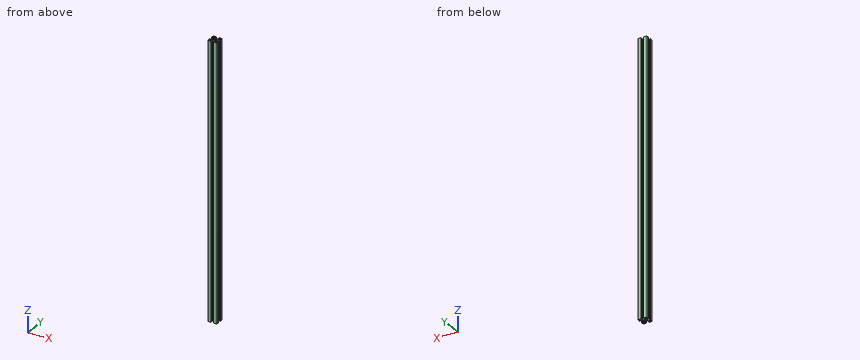
from build123d import *

# Parameters (mm, degrees)
SKETCH1_R                    = 3.52998588
BOSS_EXTRUDE1_DEPTH          = 457.2
M1_2X0_25_TAPPED_HOLE1_D     = 0.95
M1_2X0_25_TAPPED_HOLE1_DEPTH = 2.25746535


with BuildPart() as part:
    # Sketch1 → Boss-Extrude1 (new, symmetric)
    with BuildSketch(Plane.XY):
        with BuildLine():
            Line((14.49994, -4), (13.24247465, -4))
            ThreePointArc((13.24247465, -4), (12.88892126, -4.146446609), (12.74247465, -4.5))
            Line((12.74247465, -4.5), (12.74247465, -7.732519321))
            ThreePointArc((12.74247465, -7.732519321), (12.602449697, -8.097296796), (12.242781236, -8.249967))
            Line((12.242781236, -8.249967), (10.260188032, -8.249967))
            ThreePointArc((10.260188032, -8.249967), (10.068847082, -8.211906919), (9.906636056, -8.103520976))
            Line((9.906636056, -8.103520976), (5.981117769, -4.178002689))
            ThreePointArc((5.981117769, -4.178002689), (5.872731827, -4.015791664), (5.834671745, -3.824450713))
            Line((5.834671745, -3.824450713), (5.834671745, -1.01249595))
            Line((5.834671745, -1.01249595), (5.834671745, 0.88749645))
            Line((5.834671745, 0.88749645), (5.834671745, 3.824450713))
            ThreePointArc((5.834671745, 3.824450713), (5.872731827, 4.015791664), (5.981117769, 4.178002689))
            Line((5.981117769, 4.178002689), (9.906636056, 8.103520976))
            ThreePointArc((9.906636056, 8.103520976), (10.068847082, 8.211906919), (10.260188032, 8.249967))
            Line((10.260188032, 8.249967), (12.242781236, 8.249967))
            ThreePointArc((12.242781236, 8.249967), (12.602449697, 8.097296796), (12.74247465, 7.732519321))
            Line((12.74247465, 7.732519321), (12.74247465, 4.5))
            ThreePointArc((12.74247465, 4.5), (12.88892126, 4.146446609), (13.24247465, 4))
            Line((13.24247465, 4), (14.49994, 4))
            ThreePointArc((14.49994, 4), (14.853493391, 4.146446609), (14.99994, 4.5))
            Line((14.99994, 4.5), (14.99994, 12.999948))
            ThreePointArc((14.99994, 12.999948), (14.414155906, 14.414155906), (12.999948, 14.99994))
            Line((12.999948, 14.99994), (4.5, 14.99994))
            ThreePointArc((4.5, 14.99994), (4.146446609, 14.853493391), (4, 14.49994))
            Line((4, 14.49994), (4, 13.24247465))
            ThreePointArc((4, 13.24247465), (4.146446609, 12.88892126), (4.5, 12.74247465))
            Line((4.5, 12.74247465), (7.732519321, 12.74247465))
            ThreePointArc((7.732519321, 12.74247465), (8.097296796, 12.602449697), (8.249967, 12.242781236))
            Line((8.249967, 12.242781236), (8.249967, 10.260188032))
            ThreePointArc((8.249967, 10.260188032), (8.211906919, 10.068847082), (8.103520976, 9.906636056))
            Line((8.103520976, 9.906636056), (4.178002689, 5.981117769))
            ThreePointArc((4.178002689, 5.981117769), (4.015791664, 5.872731827), (3.824450713, 5.834671745))
            Line((3.824450713, 5.834671745), (0.9499962, 5.834671745))
            Line((0.9499962, 5.834671745), (-0.9499962, 5.834671745))
            Line((-0.9499962, 5.834671745), (-3.824450713, 5.834671745))
            ThreePointArc((-3.824450713, 5.834671745), (-4.015791664, 5.872731827), (-4.178002689, 5.981117769))
            Line((-4.178002689, 5.981117769), (-8.103520976, 9.906636056))
            ThreePointArc((-8.103520976, 9.906636056), (-8.211906919, 10.068847082), (-8.249967, 10.260188032))
            Line((-8.249967, 10.260188032), (-8.249967, 12.242781236))
            ThreePointArc((-8.249967, 12.242781236), (-8.097296796, 12.602449697), (-7.732519321, 12.74247465))
            Line((-7.732519321, 12.74247465), (-4.5, 12.74247465))
            ThreePointArc((-4.5, 12.74247465), (-4.146446609, 12.88892126), (-4, 13.24247465))
            Line((-4, 13.24247465), (-4, 14.49994))
            ThreePointArc((-4, 14.49994), (-4.146446609, 14.853493391), (-4.5, 14.99994))
            Line((-4.5, 14.99994), (-12.999948, 14.99994))
            ThreePointArc((-12.999948, 14.99994), (-14.414155906, 14.414155906), (-14.99994, 12.999948))
            Line((-14.99994, 12.999948), (-14.99994, 4.5))
            ThreePointArc((-14.99994, 4.5), (-14.853493391, 4.146446609), (-14.49994, 4))
            Line((-14.49994, 4), (-13.24247465, 4))
            ThreePointArc((-13.24247465, 4), (-12.88892126, 4.146446609), (-12.74247465, 4.5))
            Line((-12.74247465, 4.5), (-12.74247465, 7.732519321))
            ThreePointArc((-12.74247465, 7.732519321), (-12.602449697, 8.097296796), (-12.242781236, 8.249967))
            Line((-12.242781236, 8.249967), (-10.260188032, 8.249967))
            ThreePointArc((-10.260188032, 8.249967), (-10.068847082, 8.211906919), (-9.906636056, 8.103520976))
            Line((-9.906636056, 8.103520976), (-5.981117769, 4.178002689))
            ThreePointArc((-5.981117769, 4.178002689), (-5.872731827, 4.015791664), (-5.834671745, 3.824450713))
            Line((-5.834671745, 3.824450713), (-5.834671745, 0.88749645))
            Line((-5.834671745, 0.88749645), (-5.834671745, -1.01249595))
            Line((-5.834671745, -1.01249595), (-5.834671745, -3.824450713))
            ThreePointArc((-5.834671745, -3.824450713), (-5.872731827, -4.015791664), (-5.981117769, -4.178002689))
            Line((-5.981117769, -4.178002689), (-9.906636056, -8.103520976))
            ThreePointArc((-9.906636056, -8.103520976), (-10.068847082, -8.211906919), (-10.260188032, -8.249967))
            Line((-10.260188032, -8.249967), (-12.242781236, -8.249967))
            ThreePointArc((-12.242781236, -8.249967), (-12.602449697, -8.097296796), (-12.74247465, -7.732519321))
            Line((-12.74247465, -7.732519321), (-12.74247465, -4.5))
            ThreePointArc((-12.74247465, -4.5), (-12.88892126, -4.146446609), (-13.24247465, -4))
            Line((-13.24247465, -4), (-14.49994, -4))
            ThreePointArc((-14.49994, -4), (-14.853493391, -4.146446609), (-14.99994, -4.5))
            Line((-14.99994, -4.5), (-14.99994, -12.999948))
            ThreePointArc((-14.99994, -12.999948), (-14.414155906, -14.414155906), (-12.999948, -14.99994))
            Line((-12.999948, -14.99994), (-4.5, -14.99994))
            ThreePointArc((-4.5, -14.99994), (-4.146446609, -14.853493391), (-4, -14.49994))
            Line((-4, -14.49994), (-4, -13.24247465))
            ThreePointArc((-4, -13.24247465), (-4.146446609, -12.88892126), (-4.5, -12.74247465))
            Line((-4.5, -12.74247465), (-7.732519321, -12.74247465))
            ThreePointArc((-7.732519321, -12.74247465), (-8.097296796, -12.602449697), (-8.249967, -12.242781236))
            Line((-8.249967, -12.242781236), (-8.249967, -10.260188032))
            ThreePointArc((-8.249967, -10.260188032), (-8.211906919, -10.068847082), (-8.103520976, -9.906636056))
            Line((-8.103520976, -9.906636056), (-4.178002689, -5.981117769))
            ThreePointArc((-4.178002689, -5.981117769), (-4.015791664, -5.872731827), (-3.824450713, -5.834671745))
            Line((-3.824450713, -5.834671745), (-0.9499962, -5.834671745))
            Line((-0.9499962, -5.834671745), (0.9499962, -5.834671745))
            Line((0.9499962, -5.834671745), (3.824450713, -5.834671745))
            ThreePointArc((3.824450713, -5.834671745), (4.015791664, -5.872731827), (4.178002689, -5.981117769))
            Line((4.178002689, -5.981117769), (8.103520976, -9.906636056))
            ThreePointArc((8.103520976, -9.906636056), (8.211906919, -10.068847082), (8.249967, -10.260188032))
            Line((8.249967, -10.260188032), (8.249967, -12.242781236))
            ThreePointArc((8.249967, -12.242781236), (8.097296796, -12.602449697), (7.732519321, -12.74247465))
            Line((7.732519321, -12.74247465), (4.5, -12.74247465))
            ThreePointArc((4.5, -12.74247465), (4.146446609, -12.88892126), (4, -13.24247465))
            Line((4, -13.24247465), (4, -14.49994))
            ThreePointArc((4, -14.49994), (4.146446609, -14.853493391), (4.5, -14.99994))
            Line((4.5, -14.99994), (12.999948, -14.99994))
            ThreePointArc((12.999948, -14.99994), (14.414155906, -14.414155906), (14.99994, -12.999948))
            Line((14.99994, -12.999948), (14.99994, -4.5))
            ThreePointArc((14.99994, -4.5), (14.853493391, -4.146446609), (14.49994, -4))
        make_face()
        Circle(SKETCH1_R, mode=Mode.SUBTRACT)
        with BuildLine():
            Line((-12.6999492, -13.6999452), (-9.880960476, -13.6999452))
            ThreePointArc((-9.880960476, -13.6999452), (-9.61155387, -13.58835333), (-9.499962, -13.318946724))
            Line((-9.499962, -13.318946724), (-9.499962, -9.87996048))
            ThreePointArc((-9.499962, -9.87996048), (-9.611260978, -9.611260978), (-9.87996048, -9.499962))
            Line((-9.87996048, -9.499962), (-13.318946724, -9.499962))
            ThreePointArc((-13.318946724, -9.499962), (-13.58835333, -9.61155387), (-13.6999452, -9.880960476))
            Line((-13.6999452, -9.880960476), (-13.6999452, -12.6999492))
            ThreePointArc((-13.6999452, -12.6999492), (-13.407053153, -13.407053153), (-12.6999492, -13.6999452))
        make_face(mode=Mode.SUBTRACT)
        with BuildLine():
            Line((13.6999452, -12.6999492), (13.6999452, -9.880960476))
            ThreePointArc((13.6999452, -9.880960476), (13.58835333, -9.61155387), (13.318946724, -9.499962))
            Line((13.318946724, -9.499962), (9.87996048, -9.499962))
            ThreePointArc((9.87996048, -9.499962), (9.611260978, -9.611260978), (9.499962, -9.87996048))
            Line((9.499962, -9.87996048), (9.499962, -13.318946724))
            ThreePointArc((9.499962, -13.318946724), (9.61155387, -13.58835333), (9.880960476, -13.6999452))
            Line((9.880960476, -13.6999452), (12.6999492, -13.6999452))
            ThreePointArc((12.6999492, -13.6999452), (13.407053153, -13.407053153), (13.6999452, -12.6999492))
        make_face(mode=Mode.SUBTRACT)
        with BuildLine():
            Line((9.87996048, 9.499962), (13.318946724, 9.499962))
            ThreePointArc((13.318946724, 9.499962), (13.58835333, 9.61155387), (13.6999452, 9.880960476))
            Line((13.6999452, 9.880960476), (13.6999452, 12.6999492))
            ThreePointArc((13.6999452, 12.6999492), (13.407053153, 13.407053153), (12.6999492, 13.6999452))
            Line((12.6999492, 13.6999452), (9.880960476, 13.6999452))
            ThreePointArc((9.880960476, 13.6999452), (9.61155387, 13.58835333), (9.499962, 13.318946724))
            Line((9.499962, 13.318946724), (9.499962, 9.87996048))
            ThreePointArc((9.499962, 9.87996048), (9.611260978, 9.611260978), (9.87996048, 9.499962))
        make_face(mode=Mode.SUBTRACT)
        with BuildLine():
            Line((-13.6999452, 12.6999492), (-13.6999452, 9.880960476))
            ThreePointArc((-13.6999452, 9.880960476), (-13.58835333, 9.61155387), (-13.318946724, 9.499962))
            Line((-13.318946724, 9.499962), (-9.87996048, 9.499962))
            ThreePointArc((-9.87996048, 9.499962), (-9.611260978, 9.611260978), (-9.499962, 9.87996048))
            Line((-9.499962, 9.87996048), (-9.499962, 13.318946724))
            ThreePointArc((-9.499962, 13.318946724), (-9.61155387, 13.58835333), (-9.880960476, 13.6999452))
            Line((-9.880960476, 13.6999452), (-12.6999492, 13.6999452))
            ThreePointArc((-12.6999492, 13.6999452), (-13.407053153, 13.407053153), (-13.6999452, 12.6999492))
        make_face(mode=Mode.SUBTRACT)
    extrude(amount=BOSS_EXTRUDE1_DEPTH, both=True)

    # M1.2x0.25 Tapped Hole1
    with Locations(Plane(origin=(14.99994, 6.115, 446.77), x_dir=(0, 0, 1), z_dir=(1, 0, 0))):
        with Locations((0, 0), (0, 12.23)):
            Hole(M1_2X0_25_TAPPED_HOLE1_D / 2, depth=M1_2X0_25_TAPPED_HOLE1_DEPTH)


solid = part.part
Input: part model. Units: mm. Frame: model coordinates. Give positions to 0.01 mm unless a question says otherwise; leave off trailing zeros. Answer as a JSON object with one key per item and string values. Group by question number.
Item 1: Cut plane A-A, the plane z = 152. State how many separate pieces and enclosed holes the cut face has, and give its area (3 significant figures).
Item 2: Pin query (flat end, axial travel): P1, Ø1, axis at y = 14, z = 114, coming from the +X side; P2, Ø8, axis at x = 0, y = 0, coming from the -Z side; P3, Ø0.6, axis at y = 14, z = -131.5, coming from the -X side; P4, Ø2, axis at x = 10, y = 6, coming from the +Z side. Return the tip coordinate at first contact, or that it passes through.
Item 3: Line query: probe 1 along Y at (x, z) = (14.15, 446.77); probe 2 along Y at (x, z) = (10.5, 372.5); probe 3 along X at (y, z) = (9.75, -32). Output: solid intervals per line, ascending.
Checks:
{
 "1": {"separate pieces": "1", "enclosed holes": "5", "area": "331 mm²"},
 "2": {"P1": "stops at x = 14.94", "P2": "stops at z = -457.2", "P3": "stops at x = -14.87", "P4": "passes through"},
 "3": {"probe 1": "y = -14.64 to -6.59, -5.64 to -4, 4 to 5.64, 6.59 to 14.64", "probe 2": "y = -15 to -13.7, -9.5 to -8.25, 8.25 to 9.5, 13.7 to 15", "probe 3": "x = -15 to -13.68, -9.52 to -7.95, 7.95 to 9.52, 13.68 to 15"}
}
